```python
from build123d import *

# Parameters (mm, degrees)
SKETCH1_R           = 37.5
BOSS_EXTRUDE1_DEPTH = 5
CUT_EXTRUDE1_REACH  = 7
SKETCH2_R           = 1
CUT_EXTRUDE2_DEPTH  = 1.6
CUT_EXTRUDE3_REACH  = 7
SKETCH6_R           = 10
SKETCH7_R           = 1
CUT_EXTRUDE4_DEPTH  = 5


with BuildPart() as part:
    # Sketch1 → Boss-Extrude1 (new body)
    with BuildSketch(Plane(origin=(0, 0, 0), x_dir=(1, 0, 0), z_dir=(0, 1, 0))):
        Circle(SKETCH1_R)
    extrude(amount=-BOSS_EXTRUDE1_DEPTH)

    # Sketch2 → Cut-Extrude1 (cut, up to next)
    with BuildSketch(Plane(origin=(0, 0, 0), x_dir=(1, 0, 0), z_dir=(0, 1, 0)), mode=Mode.PRIVATE) as cut_extrude1_sk1:
        with Locations((-21.5, 0)):
            Circle(SKETCH2_R)
    cut_extrude1_tool1 = extrude(cut_extrude1_sk1.sketch, amount=-CUT_EXTRUDE1_REACH, mode=Mode.PRIVATE) & part.part
    add(cut_extrude1_tool1.solids().sort_by_distance((-21.5, 0, 0))[0], mode=Mode.SUBTRACT)
    # Sketch2 → Cut-Extrude1 (cut, up to next)
    with BuildSketch(Plane(origin=(0, 0, 0), x_dir=(1, 0, 0), z_dir=(0, 1, 0)), mode=Mode.PRIVATE) as cut_extrude1_sk2:
        with Locations((-17.393865379, 12.637382924)):
            Circle(SKETCH2_R)
    cut_extrude1_tool2 = extrude(cut_extrude1_sk2.sketch, amount=-CUT_EXTRUDE1_REACH, mode=Mode.PRIVATE) & part.part
    add(cut_extrude1_tool2.solids().sort_by_distance((-17.393865, 0, -12.637383))[0], mode=Mode.SUBTRACT)
    # Sketch2 → Cut-Extrude1 (cut, up to next)
    with BuildSketch(Plane(origin=(0, 0, 0), x_dir=(1, 0, 0), z_dir=(0, 1, 0)), mode=Mode.PRIVATE) as cut_extrude1_sk3:
        with Locations((-6.643865379, 20.4477151)):
            Circle(SKETCH2_R)
    cut_extrude1_tool3 = extrude(cut_extrude1_sk3.sketch, amount=-CUT_EXTRUDE1_REACH, mode=Mode.PRIVATE) & part.part
    add(cut_extrude1_tool3.solids().sort_by_distance((-6.643865, 0, -20.447715))[0], mode=Mode.SUBTRACT)
    # Sketch2 → Cut-Extrude1 (cut, up to next)
    with BuildSketch(Plane(origin=(0, 0, 0), x_dir=(1, 0, 0), z_dir=(0, 1, 0)), mode=Mode.PRIVATE) as cut_extrude1_sk4:
        with Locations((6.643865379, 20.4477151)):
            Circle(SKETCH2_R)
    cut_extrude1_tool4 = extrude(cut_extrude1_sk4.sketch, amount=-CUT_EXTRUDE1_REACH, mode=Mode.PRIVATE) & part.part
    add(cut_extrude1_tool4.solids().sort_by_distance((6.643865, 0, -20.447715))[0], mode=Mode.SUBTRACT)
    # Sketch2 → Cut-Extrude1 (cut, up to next)
    with BuildSketch(Plane(origin=(0, 0, 0), x_dir=(1, 0, 0), z_dir=(0, 1, 0)), mode=Mode.PRIVATE) as cut_extrude1_sk5:
        with Locations((17.393865379, 12.637382924)):
            Circle(SKETCH2_R)
    cut_extrude1_tool5 = extrude(cut_extrude1_sk5.sketch, amount=-CUT_EXTRUDE1_REACH, mode=Mode.PRIVATE) & part.part
    add(cut_extrude1_tool5.solids().sort_by_distance((17.393865, 0, -12.637383))[0], mode=Mode.SUBTRACT)
    # Sketch2 → Cut-Extrude1 (cut, up to next)
    with BuildSketch(Plane(origin=(0, 0, 0), x_dir=(1, 0, 0), z_dir=(0, 1, 0)), mode=Mode.PRIVATE) as cut_extrude1_sk6:
        with Locations((21.5, 0)):
            Circle(SKETCH2_R)
    cut_extrude1_tool6 = extrude(cut_extrude1_sk6.sketch, amount=-CUT_EXTRUDE1_REACH, mode=Mode.PRIVATE) & part.part
    add(cut_extrude1_tool6.solids().sort_by_distance((21.5, 0, 0))[0], mode=Mode.SUBTRACT)
    # Sketch2 → Cut-Extrude1 (cut, up to next)
    with BuildSketch(Plane(origin=(0, 0, 0), x_dir=(1, 0, 0), z_dir=(0, 1, 0)), mode=Mode.PRIVATE) as cut_extrude1_sk7:
        with Locations((17.393865379, -12.637382924)):
            Circle(SKETCH2_R)
    cut_extrude1_tool7 = extrude(cut_extrude1_sk7.sketch, amount=-CUT_EXTRUDE1_REACH, mode=Mode.PRIVATE) & part.part
    add(cut_extrude1_tool7.solids().sort_by_distance((17.393865, 0, 12.637383))[0], mode=Mode.SUBTRACT)
    # Sketch2 → Cut-Extrude1 (cut, up to next)
    with BuildSketch(Plane(origin=(0, 0, 0), x_dir=(1, 0, 0), z_dir=(0, 1, 0)), mode=Mode.PRIVATE) as cut_extrude1_sk8:
        with Locations((6.643865379, -20.4477151)):
            Circle(SKETCH2_R)
    cut_extrude1_tool8 = extrude(cut_extrude1_sk8.sketch, amount=-CUT_EXTRUDE1_REACH, mode=Mode.PRIVATE) & part.part
    add(cut_extrude1_tool8.solids().sort_by_distance((6.643865, 0, 20.447715))[0], mode=Mode.SUBTRACT)
    # Sketch2 → Cut-Extrude1 (cut, up to next)
    with BuildSketch(Plane(origin=(0, 0, 0), x_dir=(1, 0, 0), z_dir=(0, 1, 0)), mode=Mode.PRIVATE) as cut_extrude1_sk9:
        with Locations((-6.643865379, -20.4477151)):
            Circle(SKETCH2_R)
    cut_extrude1_tool9 = extrude(cut_extrude1_sk9.sketch, amount=-CUT_EXTRUDE1_REACH, mode=Mode.PRIVATE) & part.part
    add(cut_extrude1_tool9.solids().sort_by_distance((-6.643865, 0, 20.447715))[0], mode=Mode.SUBTRACT)
    # Sketch2 → Cut-Extrude1 (cut, up to next)
    with BuildSketch(Plane(origin=(0, 0, 0), x_dir=(1, 0, 0), z_dir=(0, 1, 0)), mode=Mode.PRIVATE) as cut_extrude1_sk10:
        with Locations((-17.393865379, -12.637382924)):
            Circle(SKETCH2_R)
    cut_extrude1_tool10 = extrude(cut_extrude1_sk10.sketch, amount=-CUT_EXTRUDE1_REACH, mode=Mode.PRIVATE) & part.part
    add(cut_extrude1_tool10.solids().sort_by_distance((-17.393865, 0, 12.637383))[0], mode=Mode.SUBTRACT)

    # Sketch4 → Cut-Extrude2 (cut)
    with BuildSketch(Plane.XZ.offset(5)):
        Polygon((-15.525520661, 11.27995103), (-15.284122516, 13.576700966), (-17.152467233, 14.93413286), (-19.262210097, 13.994814819), (-19.503608243, 11.698064883), (-17.635263525, 10.340632988), align=None)
        Polygon((-19.190598923, 0), (-20.345299462, 2), (-22.654700538, 2), (-23.809401077, 0), (-22.654700538, -2), (-20.345299462, -2), align=None)
        Polygon((-5.9302212, 18.251344158), (-4.384930257, 19.967563618), (-5.098574436, 22.16393456), (-7.357509559, 22.644086043), (-8.902800501, 20.927866583), (-8.189156322, 18.73149564), align=None)
        Polygon((5.9302212, 18.251344158), (8.189156322, 18.73149564), (8.902800501, 20.927866583), (7.357509559, 22.644086043), (5.098574436, 22.16393456), (4.384930257, 19.967563618), align=None)
        Polygon((15.525520661, 11.27995103), (17.635263525, 10.340632988), (19.503608243, 11.698064883), (19.262210097, 13.994814819), (17.152467233, 14.93413286), (15.284122516, 13.576700966), align=None)
        Polygon((19.190598923, 0), (20.345299462, -2), (22.654700538, -2), (23.809401077, 0), (22.654700538, 2), (20.345299462, 2), align=None)
        Polygon((15.525520661, -11.27995103), (15.284122516, -13.576700966), (17.152467233, -14.93413286), (19.262210097, -13.994814819), (19.503608243, -11.698064883), (17.635263525, -10.340632988), align=None)
        Polygon((5.9302212, -18.251344158), (4.384930257, -19.967563618), (5.098574436, -22.16393456), (7.357509559, -22.644086043), (8.902800501, -20.927866583), (8.189156322, -18.73149564), align=None)
        Polygon((-5.9302212, -18.251344158), (-8.189156322, -18.73149564), (-8.902800501, -20.927866583), (-7.357509559, -22.644086043), (-5.098574436, -22.16393456), (-4.384930257, -19.967563618), align=None)
        Polygon((-15.525520661, -11.27995103), (-17.635263525, -10.340632988), (-19.503608243, -11.698064883), (-19.262210097, -13.994814819), (-17.152467233, -14.93413286), (-15.284122516, -13.576700966), align=None)
    extrude(amount=-CUT_EXTRUDE2_DEPTH, mode=Mode.SUBTRACT)

    # Sketch6 → Cut-Extrude3 (cut, up to next)
    with BuildSketch(Plane(origin=(0, 0, 0), x_dir=(1, 0, 0), z_dir=(0, 1, 0)), mode=Mode.PRIVATE) as cut_extrude3_sk1:
        Circle(SKETCH6_R)
    cut_extrude3_tool1 = extrude(cut_extrude3_sk1.sketch, amount=-CUT_EXTRUDE3_REACH, mode=Mode.PRIVATE) & part.part
    add(cut_extrude3_tool1.solids().sort_by_distance((0, 0, 0))[0], mode=Mode.SUBTRACT)

    # Sketch7 → Cut-Extrude4 (cut)
    with BuildSketch(Plane(origin=(0, 0, 0), x_dir=(1, 0, 0), z_dir=(0, 1, 0))):
        with Locations((0, -34.458998708)):
            Circle(SKETCH7_R)
        with Locations((-29.84236827, 17.229499354)):
            Circle(SKETCH7_R)
        with Locations((29.84236827, 17.229499354)):
            Circle(SKETCH7_R)
    extrude(amount=-CUT_EXTRUDE4_DEPTH, mode=Mode.SUBTRACT)


solid = part.part
```
Read the model definition and answer for the solid it produces. Units are mm, in the model's axes. A direction names the side the tool comes from. Give positions to 0.01 mm unless a question says otherwise; leave off trailing zeros. Write each loop counter-clockwise with the first axis right and the second up, starting at its lowest first coordinate (ties: lowest second). Pieces come first, ordered by that corner, then holes. Notation, with made-up numbers: (28, 32.5) -> (79, 32.5) arc R29 cw to (79, 64.5) -> close; hole circle Ø4 at (-11.5, -36.75). An arc over 180 degrees is marked (long way). Answer in a Markdown table with one row per item.
1) Section D-D on y = -1.4 is taken. Count the separate pieces of the cut face and the enclosed holes in it, plus the area to 3 significant figures.
Results list:
| item | result |
|---|---|
| separate pieces | 1 |
| enclosed holes | 14 |
| area | 4,060 mm^2 |
2) Each of these flat-tipped pins is pushed along its axis until it touches: pin 1 Ø0.8 at (x, y) = (21, -4.5) entering from -Z; pin 2 Ø2.5 at (x, z) = (17.39, 12.64) entering from -Y; pin 3 Ø2 at (y, z) = (-4, 24) entering from +X. Where does it stop, or does it pass through?
Results list:
| item | result |
|---|---|
| pin 1 | z = -31.34 |
| pin 2 | y = -3.4 |
| pin 3 | x = 29.62 |
3) Straight lines are drawn through the part: line 1 (X direction, y = -2.9, z = 0); line 2 (X direction, y = -3.5, z = 0); line 3 (X direction, y = -3.85, z = 19). For each, find the intervals that lie inside material, in ascending order. Write a range as [from, to].
Results list:
| item | result |
|---|---|
| line 1 | [-37.5, -22.5], [-20.5, -10], [10, 20.5], [22.5, 37.5] |
| line 2 | [-37.5, -23.81], [-19.19, -10], [10, 19.19], [23.81, 37.5] |
| line 3 | [-32.33, -8.28], [-5.26, 5.26], [8.28, 32.33] |
4) Section C-C on z = 6 is taken. Give the vertices of the cut face in (x, y).
Results list:
| item | result |
|---|---|
| outline | (-37.02, -5) -> (-8, -5) -> (-8, 0) -> (-37.02, 0) -> close; (8, -5) -> (37.02, -5) -> (37.02, 0) -> (8, 0) -> close |
5) Section A-A on x = 0 is taken. Give the vertices of the cut face in (y, z), plus the area to 3 significant figures.
Results list:
| item | result |
|---|---|
| outline | (-5, -37.5) -> (0, -37.5) -> (0, -10) -> (-5, -10) -> close; (-5, 10) -> (0, 10) -> (0, 33.46) -> (-5, 33.46) -> close; (-5, 35.46) -> (0, 35.46) -> (0, 37.5) -> (-5, 37.5) -> close |
| area | 265 mm^2 |
6) Determine the mould class of faces 3 (the flat face through (18.22, -4.21, 14.46)), 4 (the flat face through (8, 0, 8)) for opening direction X: released by +X, released by -X, zero draft, split by the parting line, or undercut.
Results list:
| item | result |
|---|---|
| face 3 | undercut |
| face 4 | zero draft |
7) A tool of negligible diameter and unlimited length cuts with its end or side. For faces 1 (the flat face through (8, -5, 8)), 2 (the flat face through (6.2, -4.2, 22.4)), from which of +Z, -Z, +X, -X, +Y, -Y can it reach the whole face along a straight path? Write none if from no direction.
Results list:
| item | result |
|---|---|
| face 1 | +Z, -Z, +X, -X, -Y |
| face 2 | -Y |
8) Section B-B on x = 21.5 is taken. Give the vertices of the cut face in (y, z), plus the area to 3 significant figures.
Results list:
| item | result |
|---|---|
| outline | (-5, -30.72) -> (0, -30.72) -> (0, -1) -> (-3.4, -1) -> (-3.4, -2) -> (-5, -2) -> close; (-5, 2) -> (-3.4, 2) -> (-3.4, 1) -> (0, 1) -> (0, 30.72) -> (-5, 30.72) -> close |
| area | 294 mm^2 |
